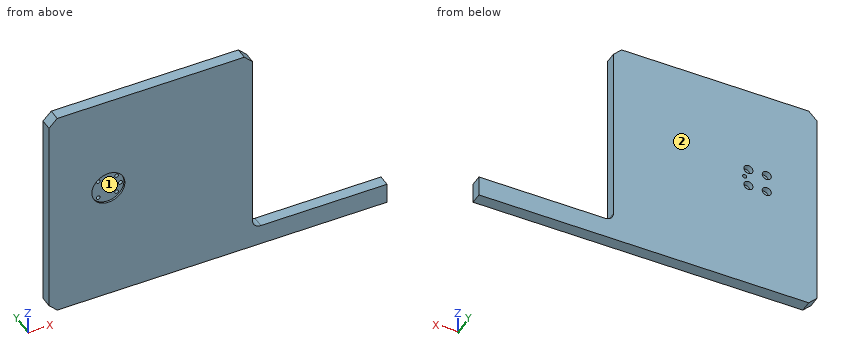
from build123d import *

# Parameters (mm, degrees)
BOSS_EXTRUDE1_DEPTH                                 = 14
SKETCH2_R                                           = 20
CUT_EXTRUDE1_DEPTH                                  = 2.28
CBORE_FOR_00_BINDING_HEAD_MACHINE_SCREW_D           = 4.499991
CBORE_FOR_00_BINDING_HEAD_MACHINE_SCREW_CBORE_D     = 11.0000034
CBORE_FOR_00_BINDING_HEAD_MACHINE_SCREW_CBORE_DEPTH = 7.0000114
SKETCH5_R                                           = 2.5
CUT_EXTRUDE2_DEPTH                                  = 369.713712791


with BuildPart() as part:
    # Sketch1 → Boss-Extrude1 (new body)
    with BuildSketch(Plane(origin=(0, 0, 0), x_dir=(1, 0, 0), z_dir=(0, 1, 0))):
        with BuildLine():
            Line((337.94, 147), (337.94, 122))
            Line((337.94, 122), (184.94, 122))
            ThreePointArc((184.94, 122), (177.868932188, 119.071067812), (174.94, 112))
            Line((174.94, 112), (174.94, -110))
            Line((174.94, -110), (164.94, -120))
            Line((164.94, -120), (-62.06, -120))
            Line((-62.06, -120), (-72.06, -110))
            Line((-72.06, -110), (-72.06, 137))
            Line((-72.06, 137), (-62.06, 147))
            Line((-62.06, 147), (337.94, 147))
        make_face()
    extrude(amount=BOSS_EXTRUDE1_DEPTH)

    # Sketch2 → Cut-Extrude1 (cut)
    with BuildSketch(Plane(origin=(0, 0, 0), x_dir=(1, 0, 0), z_dir=(0, 1, 0))):
        with Locations(Location((0, 0, 0), (0, 0, 90))):
            Circle(SKETCH2_R)
    extrude(amount=CUT_EXTRUDE1_DEPTH, mode=Mode.SUBTRACT)

    # CBORE for #00 Binding Head Machine Screw1 (through all)
    with Locations(Plane(origin=(0, 14, 0), x_dir=(-1, 0, 0), z_dir=(0, 1, 0))):
        with Locations((11.136931804, 11.136931804), (-11.136931804, 11.136931804), (-11.136931804, -11.136931804), (11.136931804, -11.136931804)):
            CounterBoreHole(CBORE_FOR_00_BINDING_HEAD_MACHINE_SCREW_D / 2, CBORE_FOR_00_BINDING_HEAD_MACHINE_SCREW_CBORE_D / 2, CBORE_FOR_00_BINDING_HEAD_MACHINE_SCREW_CBORE_DEPTH)

    # Sketch5 → Cut-Extrude2 (cut, through all)
    with BuildSketch(Plane(origin=(0, 2.28, 0), x_dir=(-1, 0, 0), z_dir=(0, -1, 0))):
        with Locations(Location((-15.75, 0, 0), (0, 0, 90))):
            Circle(SKETCH5_R)
    extrude(amount=-CUT_EXTRUDE2_DEPTH, mode=Mode.SUBTRACT)


solid = part.part
The listing builds one solid part. Answer for the finished solid, in the listing's coordinates (mm). Face numbers are marked on the shaded views. Give positions to 0.01 mm unless a question says otherwise; leave off trailing zeros. Order: outer loops, then holes, each group sorted by start corner. A loop starts at its lowest first (then second) coordinate and runs counter-clockwise, first axis right, second up. Notation, with made-up numbers: (-20, -26) -> (-14, -26) arc R13 cw to (-14, -18) -> close; hole circle Ø10 at (-21, -28). An arc over 180 degrees is marked (long way). Put each result on its own line as item: value.
Item 1: Straight lines are drawn through the part: line 1 (X direction, y = 8.75, z = 38); line 2 (X direction, y = 12.25, z = -1); line 3 (Z direction, x = 200, y = 3). For each, find the intervals that lie inside material, in ascending order.
Established:
line 1: x = -72.06 to 174.94
line 2: x = -72.06 to 13.46, 18.04 to 174.94
line 3: z = -147 to -122
Item 2: For a pull along Z with two mould halves and no side action, classify the marked faces 1 and 2 as released by +Z, released by -Z, zero draft, split by the parting line, or undercut.
Established:
face 1: undercut
face 2: zero draft
Item 3: Given P1, Ø4, axis at x = 248.5, y = 6, coming from the +Z side; P2, Ø7, axis at x = -11.14, z = 11.14, coming from the +Y side; P3, Ø5, axis at y = 7.5, z = -101, coming from the +X side, each flat-ended and moving along its own axis, determine where each tip first touches the part or whether it passes through.
Established:
P1: stops at z = -122
P2: stops at y = 7
P3: stops at x = 174.94
Item 4: A cutting plane is placed at B-B on x = 292.5. Give the vertices of the cut face in (y, z).
Established:
outline: (0, -147) -> (14, -147) -> (14, -122) -> (0, -122) -> close
Item 5: A cutting plane is placed at A-A on x = 0. Give the vertices of the cut face in (y, z).
Established:
outline: (0, -147) -> (14, -147) -> (14, 120) -> (0, 120) -> (0, 20) -> (2.28, 20) -> (2.28, -20) -> (0, -20) -> close
